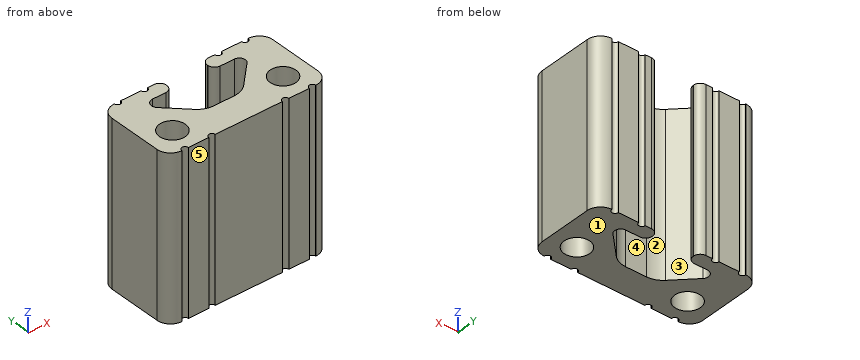
```python
from build123d import *

# Parameters (mm, degrees)
SKETCH1_R      = 2.032
EXTRUDE1_DEPTH = 25.4


with BuildPart() as part:
    # Sketch1 → Extrude1 (new body)
    with BuildSketch(Plane.XY):
        with BuildLine():
            Line((9.551093887, 6.35), (6.330982008, 6.35))
            ThreePointArc((6.330982008, 6.35), (5.824379679, 5.843397671), (5.31777735, 6.35))
            Line((5.31777735, 6.35), (4.28752, 6.35))
            ThreePointArc((4.28752, 6.35), (3.545750844, 6.042749156), (3.2385, 5.30098))
            Line((3.2385, 5.30098), (3.2385, 5.18922))
            ThreePointArc((3.2385, 5.18922), (3.545750844, 4.447450844), (4.28752, 4.1402))
            Line((4.28752, 4.1402), (6.541264932, 4.1402))
            ThreePointArc((6.541264932, 4.1402), (7.403778411, 3.563601238), (7.200674335, 2.54618079))
            Line((7.200674335, 2.54618079), (3.874487735, -0.773919123))
            ThreePointArc((3.874487735, -0.773919123), (2.845157282, -1.460673567), (1.631480681, -1.7018))
            Line((1.631480681, -1.7018), (-1.631480681, -1.7018))
            ThreePointArc((-1.631480681, -1.7018), (-2.845157282, -1.460673567), (-3.874487735, -0.773919123))
            Line((-3.874487735, -0.773919123), (-7.091634343, 2.437340333))
            ThreePointArc((-7.091634343, 2.437340333), (-7.30860647, 3.524230776), (-6.387200124, 4.1402))
            Line((-6.387200124, 4.1402), (-4.28752, 4.1402))
            ThreePointArc((-4.28752, 4.1402), (-3.545750844, 4.447450844), (-3.2385, 5.18922))
            Line((-3.2385, 5.18922), (-3.2385, 5.30098))
            ThreePointArc((-3.2385, 5.30098), (-3.545750844, 6.042749156), (-4.28752, 6.35))
            Line((-4.28752, 6.35), (-5.319235427, 6.35))
            ThreePointArc((-5.319235427, 6.35), (-5.825837756, 5.843397671), (-6.332440085, 6.35))
            Line((-6.332440085, 6.35), (-9.552501021, 6.35))
            ThreePointArc((-9.552501021, 6.35), (-10.056951984, 5.843402239), (-10.565687406, 6.345697309))
            Line((-10.565687406, 6.345697309), (-10.590059723, 6.345701253))
            ThreePointArc((-10.590059723, 6.345701253), (-12.083428447, 5.727229281), (-12.7, 4.233074923))
            Line((-12.7, 4.233074923), (-12.7, -4.233074923))
            ThreePointArc((-12.7, -4.233074923), (-12.072915167, -5.733409532), (-10.564685825, -6.341261141))
            ThreePointArc((-10.564685825, -6.341261141), (-10.053713904, -5.834598435), (-9.551557924, -6.35))
            Line((-9.551557924, -6.35), (-6.323021107, -6.35))
            ThreePointArc((-6.323021107, -6.35), (-5.816495529, -5.83457959), (-5.309969951, -6.35))
            Line((-5.309969951, -6.35), (5.309969951, -6.35))
            ThreePointArc((5.309969951, -6.35), (5.816495529, -5.83457959), (6.323021107, -6.35))
            Line((6.323021107, -6.35), (9.550160942, -6.35))
            ThreePointArc((9.550160942, -6.35), (10.051855758, -5.834602622), (10.563288148, -6.340338775))
            Line((10.563288148, -6.340338775), (10.589922543, -6.34049468))
            ThreePointArc((10.589922543, -6.34049468), (12.081868228, -5.723579066), (12.7, -4.23213684))
            Line((12.7, -4.23213684), (12.7, 4.244714967))
            ThreePointArc((12.7, 4.244714967), (12.082100067, 5.735925507), (10.590578068, 6.353073239))
            Line((10.590578068, 6.353073239), (10.564289268, 6.353065837))
            ThreePointArc((10.564289268, 6.353065837), (10.059229141, 5.84339999), (9.551093887, 6.35))
        make_face()
        with Locations((8.7376, -2.3876)):
            Circle(SKETCH1_R, mode=Mode.SUBTRACT)
        with Locations((-8.7376, -2.3876)):
            Circle(SKETCH1_R, mode=Mode.SUBTRACT)
    extrude(amount=-EXTRUDE1_DEPTH)


solid = part.part
```
Can you work these out from the model? Positions are in its coordinate system, mm. Face numbers are marked on the shaded views. A direction names the side the tool comes from. Coordinates: 2 decimals unless noted, no trailing zeros. Loops run counter-clockwise (first coordinate to the right, second up) from the corner with the lowest first, then second, coordinate; pieces in that order, holes last. Notation, with made-up numbers: (87, -25.75) - (93, -25.75) arc R16 ccw to (93, -12.75) - close; hole circle Ø6 at (56.25, -4). An arc over 180 degrees is marked (long way). Use a Markdown table: item, result.
Item 1: I want a section at C-C on z = -3.75. Give the number of separate pieces and of enclosed holes in the cut face, and give its area (3 significant figures).
Numbers:
| item | result |
|---|---|
| separate pieces | 1 |
| enclosed holes | 2 |
| area | 208 mm2 |
Item 2: If I drill on probe 1 along X at (y, z) = (-3.75, -18.75); probe 2 along X at (y, z) = (-3.25, -21); probe 3 along X at (y, z) = (3.25, -20.75), over which ranges is the centre line in solid material (lowest first)? Write a range as from..to.
Numbers:
| item | result |
|---|---|
| probe 1 | x = -12.7..-10.25, -7.23..7.23, 10.25..12.7 |
| probe 2 | x = -12.7..-10.58, -6.9..6.9, 10.58..12.7 |
| probe 3 | x = -12.7..-7.38, 7.47..12.7 |
Item 3: For the marked faces 1 and 2, which set-ups out of +Z, -Z, +X, -X, +Y, -Y let a thin tool reach every point of the face, with its end or its side?
Numbers:
| item | result |
|---|---|
| face 1 | -Z, +X, -X, +Y, -Y |
| face 2 | +Z, -Z |
Item 4: Will these pins go through, and if not, where does the flat tip stop? pin 1 (3.5 mm diameter, centred on x = -7.5, z = -13.5, fed in from +Y); pin 2 (3 mm diameter, centred on x = 0.5, z = -17, fed in from +Y).
Numbers:
| item | result |
|---|---|
| pin 1 | stops at y = 6.35 |
| pin 2 | stops at y = -1.68 |
Item 5: I want a section at A-A on x = 8. Please give me the cut outline in (y, z).
Numbers:
| item | result |
|---|---|
| outline | (-6.35, -25.4) - (-4.28, -25.4) - (-4.28, 0) - (-6.35, 0) - close; (-0.49, -25.4) - (6.35, -25.4) - (6.35, 0) - (-0.49, 0) - close |
Item 6: I want a section at B-B on y = 1.25. Please give me the cut outline in (x, z), and give its area (3 significant figures).
Numbers:
| item | result |
|---|---|
| outline | (-12.7, -25.4) - (-5.9, -25.4) - (-5.9, 0) - (-12.7, 0) - close; (5.9, -25.4) - (12.7, -25.4) - (12.7, 0) - (5.9, 0) - close |
| area | 345 mm2 |
Item 7: We'd pull the mould along Y, two halves only. Please class the marked faces 3, 4 and 5: released by +Y, released by -Y, zero draft, split by the parting line, or undercut.
Numbers:
| item | result |
|---|---|
| face 3 | undercut |
| face 4 | released by +Y |
| face 5 | released by -Y |
Item 8: I want a section at D-D on y = -5.25. Please give me the cut outline in (x, z).
Numbers:
| item | result |
|---|---|
| outline | (-12.44, -25.4) - (12.44, -25.4) - (12.44, 0) - (-12.44, 0) - close |
